from build123d import *

# Parameters (mm, degrees)
F0_W     = 45
F0_H     = 24
F0_R     = 2.75
F1_DEPTH = 15
F2_R     = 6
F2_R_2   = 2.75
F3_DEPTH = 12
F4_R     = 2.75
F5_DEPTH = 24.001


with BuildPart() as f1:
    # F0 (on Top) → F1 (new body)
    with BuildSketch(Plane.XY):
        Rectangle(F0_W, F0_H)
        with Locations((-10, 0)):
            Circle(F0_R, mode=Mode.SUBTRACT)
        with Locations((10, 0)):
            Circle(F0_R, mode=Mode.SUBTRACT)
    extrude(amount=F1_DEPTH)

    # F2 (on face) → F3 (cut)
    with BuildSketch(Plane.XY.offset(15)):
        with Locations((-10, 0)):
            Circle(F2_R)
        with Locations((-10, 0)):
            Circle(F2_R_2, mode=Mode.SUBTRACT)
        with Locations((10, 0)):
            Circle(F2_R)
        with Locations((10, 0)):
            Circle(F2_R_2, mode=Mode.SUBTRACT)
    extrude(amount=-F3_DEPTH, mode=Mode.SUBTRACT)

    # F4 (on face) → F5 (cut, through all)
    with BuildSketch(Plane.XZ.offset(12)):
        with Locations((0, 9)):
            Circle(F4_R)
        with BuildLine():
            ThreePointArc((-2.774851, 13.159351), (0, 14), (2.774851, 13.159351))
            Line((2.774851, 13.159351), (22.5, 0))
            Line((22.5, 0), (22.5, 15))
            Line((22.5, 15), (-22.5, 15))
            Line((-22.5, 15), (-22.5, 0))
            Line((-22.5, 0), (-2.774851, 13.159351))
        make_face()
    extrude(amount=-F5_DEPTH, mode=Mode.SUBTRACT)


solid = f1.part
Could you check a few things on this model? Use its own coordinates, in mm. A direction names the side the tool comes from. Give positions to 0.01 mm unless a question says otherwise; leave off trailing zeros. Order: outer loops, then holes, each group sorted by start corner. A loop starts at its lowest first (then second) coordinate and runs counter-clockwise, first axis right, second up.
1. Suppose I cut it at D-D (z = 1). List the corners of the cut face in (x, y) for me.
2. Suppose I cut it at A-A (x = 0). List the corners of the cut face in (y, z) for me, plus the area to 3 significant figures.
3. For faces 5 (the cylindrical face through (-4.277, 1.802, 6.698)), 6 (the flat face through (0, -12, 4)), which set-ups out of +Z, -Z, +X, -X, +Y, -Y let a thin tool reach every point of the face, with its end or its side?
4. Suppose I cut it at B-B (y = 0). List the corners of the cut face in (x, z) for me, plus the area to 3 significant figures.
5. We'd pull the mould along Y, two halves only. Please class faces 1 (the flat face through (-17.159, -0.168, 3.563)), 2 (the flat face through (13, -1, 3)), 3 (the flat face through (0, 12, 4)), 4 (the cylindrical face through (4, 0, 7)): pulls with the +Y half, pulls with the -Y half, needs draft (parallel to the pull), parting line crosses it, or undercut.
6. Will these pins go through, and if not, where does the flat tip stop? P1, Ø9.5, axis at x = 10, y = 0, coming from the +Z side; P2, Ø1, axis at x = -15.5, y = 2, coming from the +Z side; P3, Ø5, axis at y = 0.5, z = 10, coming from the -X side.
7. Suppose I cut it at C-C (y = -9.5). List the corners of the cut face in (x, z) for me, plus the area to 3 significant figures.
8. I need wall thicknesses on L1, parallel to Y at x = 10, z = 2.15; L2, parallel to X at y = -2, z = 2.5; L3, parallel to Z at x = 9.5, y = 3.25. Which ranges of each line are inside material? Lowest first, please.
Solved:
1. outline: (-21, -12) - (21, -12) - (21, 12) - (-21, 12) - close; hole circle Ø5.5 at (-10, 0); hole circle Ø5.5 at (10, 0)
2. outline: (-12, 0) - (12, 0) - (12, 6.25) - (-12, 6.25) - close; (-12, 11.75) - (12, 11.75) - (12, 14) - (-12, 14) - close
2. area: 204 mm2
3. face 5: +Z
3. face 6: +Z, -Z, +X, -X, -Y
4. outline: (-22.5, 0) - (-12.75, 0) - (-12.75, 3) - (-16, 3) - (-16, 4.34) - close; (-7.25, 0) - (7.25, 0) - (7.25, 3) - (4, 3) - (4, 12.34) - (2.77, 13.16) arc R5 ccw to (-2.77, 13.16) - (-4, 12.34) - (-4, 3) - (-7.25, 3) - close; (12.75, 0) - (22.5, 0) - (16, 4.34) - (16, 3) - (12.75, 3) - close; hole circle Ø5.5 at (0, 9)
4. area: 151 mm2
5. face 1: needs draft
5. face 2: undercut
5. face 3: pulls with the +Y half
5. face 4: undercut
6. P1: stops at z = 3
6. P2: stops at z = 4.7
6. P3: stops at x = -4.8
7. outline: (-22.5, 0) - (22.5, 0) - (2.77, 13.16) arc R5 ccw to (-2.77, 13.16) - close; hole circle Ø5.5 at (0, 9)
7. area: 312 mm2
8. L1: y = -12 to -2.75, 2.75 to 12
8. L2: x = -18.75 to -11.89, -8.11 to 8.11, 11.89 to 18.75
8. L3: z = 0 to 3
